```python
from build123d import *

# Parameters (mm, degrees)
SKETCH1_W                = 240
SKETCH1_H                = 151
BOSS_EXTRUDE1_DEPTH      = 5
SKETCH5_R                = 2
CUT_EXTRUDE1_DEPTH       = 5
SKETCH6_R                = 4
SKETCH6_R_2              = 2
BOSS_EXTRUDE2_DEPTH      = 5
CUT_EXTRUDE2_DEPTH       = 5
SKETCH8_W                = 30
SKETCH8_H                = 12.5
CUT_EXTRUDE3_DEPTH       = 5
SKETCH9_W                = 59
SKETCH9_H                = 121
CUT_EXTRUDE4_DEPTH       = 5
SKETCH12_W               = 18
SKETCH12_H               = 40
CUT_EXTRUDE7_DEPTH       = 10
SKETCH15_R               = 2
CUT_EXTRUDE9_DEPTH       = 5
SKETCH16_W               = 5.2
SKETCH16_H               = 20.2
CUT_EXTRUDE10_DEPTH      = 5
CUT_EXTRUDE11_DEPTH      = 10
CUT_EXTRUDE13_DEPTH      = 143.667445481
CUT_EXTRUDE13_DEPTH_BACK = 10
SKETCH23_R               = 2
CUT_EXTRUDE16_DEPTH      = 5
SKETCH24_R               = 4
SKETCH24_R_2             = 2
BOSS_EXTRUDE4_DEPTH      = 5
CUT_EXTRUDE19_DEPTH      = 10
SKETCH32_W               = 4
SKETCH32_H               = 30
SKETCH32_H_2             = 15
BOSS_EXTRUDE6_DEPTH      = 5
FILLET1_R                = 5
FILLET2_R                = 2
CUT_EXTRUDE22_DEPTH      = 5
SKETCH37_R               = 2
CUT_EXTRUDE25_DEPTH      = 10
SKETCH38_R               = 2
CUT_EXTRUDE26_DEPTH      = 10
CUT_EXTRUDE29_DEPTH      = 10
SKETCH43_R               = 2
CUT_EXTRUDE30_DEPTH      = 10
SKETCH44_R               = 4
SKETCH44_R_2             = 2
BOSS_EXTRUDE7_DEPTH      = 5
CUT_EXTRUDE31_DEPTH      = 10
CUT_EXTRUDE32_DEPTH      = 10
SKETCH47_R               = 2
CUT_EXTRUDE33_DEPTH      = 10
SKETCH48_W               = 15
SKETCH48_H               = 5
CUT_EXTRUDE34_DEPTH      = 5


with BuildPart() as part:
    # Sketch1 → Boss-Extrude1 (new body)
    with BuildSketch(Plane.XY):
        Rectangle(SKETCH1_W, SKETCH1_H)
    extrude(amount=BOSS_EXTRUDE1_DEPTH)

    # Sketch5 → Cut-Extrude1 (cut)
    with BuildSketch(Plane(origin=(0, 0, 0), x_dir=(-1, 0, 0), z_dir=(0, 0, -1))):
        with Locations((35.2, -73)):
            Circle(SKETCH5_R)
        with Locations((79.8, -73)):
            Circle(SKETCH5_R)
        with Locations((22.5, -65.3)):
            Circle(SKETCH5_R)
        with Locations(Location((22.5, -20.7, 0), (0, 0, 180))):
            Circle(SKETCH5_R)
        with Locations(Location((79.8, -13, 0), (0, 0, 180))):
            Circle(SKETCH5_R)
        with Locations(Location((35.2, -13, 0), (0, 0, 180))):
            Circle(SKETCH5_R)
    extrude(amount=-CUT_EXTRUDE1_DEPTH, mode=Mode.SUBTRACT)

    # Sketch6 → Boss-Extrude2 (add)
    # profile 1 of 2: a face of its own
    with BuildSketch(Plane(origin=(0, 0, 0), x_dir=(-1, 0, 0), z_dir=(0, 0, -1))):
        with Locations((35.2, -73)):
            Circle(SKETCH6_R)
        with Locations((35.2, -73)):
            Circle(SKETCH6_R_2, mode=Mode.SUBTRACT)
    # profile 2 of 2: a face of its own
    with BuildSketch(Plane(origin=(0, 0, 0), x_dir=(-1, 0, 0), z_dir=(0, 0, -1))):
        with Locations((79.8, -73)):
            Circle(SKETCH6_R)
        with Locations((79.8, -73)):
            Circle(SKETCH6_R_2, mode=Mode.SUBTRACT)
    extrude(amount=-BOSS_EXTRUDE2_DEPTH)

    # Sketch7 → Cut-Extrude2 (cut)
    with BuildSketch(Plane(origin=(0, 0, 0), x_dir=(-1, 0, 0), z_dir=(0, 0, -1))):
        with BuildLine():
            Line((120, -63), (43.5, -63))
            ThreePointArc((43.5, -63), (23.5, -43), (43.5, -23))
            Line((43.5, -23), (120, -23))
            Line((120, -23), (120, -63))
        make_face()
    extrude(amount=-CUT_EXTRUDE2_DEPTH, mode=Mode.SUBTRACT)

    # Sketch8 → Cut-Extrude3 (cut)
    with BuildSketch(Plane(origin=(0, 0, 0), x_dir=(-1, 0, 0), z_dir=(0, 0, -1))):
        with Locations((105, -69.25)):
            Rectangle(SKETCH8_W, SKETCH8_H)
    extrude(amount=-CUT_EXTRUDE3_DEPTH, mode=Mode.SUBTRACT)

    # Sketch9 → Cut-Extrude4 (cut)
    with BuildSketch(Plane(origin=(0, 0, 0), x_dir=(-1, 0, 0), z_dir=(0, 0, -1))):
        with Locations((-90.5, -15)):
            Rectangle(SKETCH9_W, SKETCH9_H)
    extrude(amount=-CUT_EXTRUDE4_DEPTH, mode=Mode.SUBTRACT)

    # Sketch12 → Cut-Extrude7 (cut)
    with BuildSketch(Plane(origin=(0, 0, 0), x_dir=(-1, 0, 0), z_dir=(0, 0, -1))):
        with Locations((-3, 55.5)):
            Rectangle(SKETCH12_W, SKETCH12_H)
    extrude(amount=-CUT_EXTRUDE7_DEPTH, mode=Mode.SUBTRACT)

    # Sketch15 → Cut-Extrude9 (cut)
    with BuildSketch(Plane.XY.offset(5)):
        with Locations((-63.5, 68.3)):
            Circle(SKETCH15_R)
    extrude(amount=-CUT_EXTRUDE9_DEPTH, mode=Mode.SUBTRACT)

    # Sketch16 → Cut-Extrude10 (cut)
    with BuildSketch(Plane(origin=(0, 0, 0), x_dir=(-1, 0, 0), z_dir=(0, 0, -1))):
        with Locations((63.6, 35.6)):
            Rectangle(SKETCH16_W, SKETCH16_H)
    extrude(amount=-CUT_EXTRUDE10_DEPTH, mode=Mode.SUBTRACT)

    # Sketch18 → Cut-Extrude11 (cut)
    with BuildSketch(Plane(origin=(0, 0, 0), x_dir=(-1, 0, 0), z_dir=(0, 0, -1))):
        with BuildLine():
            Line((-2.007007892, 12.8501367), (-2.007007892, 2.8501367))
            ThreePointArc((-2.007007892, 2.8501367), (-9.507007892, -4.6498633), (-17.007007892, 2.8501367))
            Line((-17.007007892, 2.8501367), (-17.007007892, 12.8501367))
            ThreePointArc((-17.007007892, 12.8501367), (-9.507007892, 20.3501367), (-2.007007892, 12.8501367))
        make_face()
    extrude(amount=-CUT_EXTRUDE11_DEPTH, mode=Mode.SUBTRACT)

    # Sketch20 → Cut-Extrude13 (cut, two sides: drawn at the far end of the back side and taken through both)
    with BuildSketch(Plane(origin=(0, 0, 0), x_dir=(-1, 0, 0), z_dir=(0, 0, -1)).offset(-CUT_EXTRUDE13_DEPTH_BACK)):
        with BuildLine():
            ThreePointArc((-33.7955627, -69.5), (-42.0455627, -61.25), (-50.2955627, -69.5))
            Line((-50.2955627, -69.5), (-50.2955627, -75.5))
            Line((-50.2955627, -75.5), (-33.7955627, -75.5))
            Line((-33.7955627, -75.5), (-33.7955627, -69.5))
        make_face()
    extrude(amount=CUT_EXTRUDE13_DEPTH + CUT_EXTRUDE13_DEPTH_BACK, mode=Mode.SUBTRACT)

    # Sketch23 → Cut-Extrude16 (cut)
    with BuildSketch(Plane(origin=(0, 0, 0), x_dir=(-1, 0, 0), z_dir=(0, 0, -1))):
        with Locations((-107.8, 73)):
            Circle(SKETCH23_R)
        with Locations((-30.2, 73)):
            Circle(SKETCH23_R)
    extrude(amount=-CUT_EXTRUDE16_DEPTH, mode=Mode.SUBTRACT)

    # Sketch24 → Boss-Extrude4 (add)
    # profile 1 of 2: a face of its own
    with BuildSketch(Plane(origin=(0, 0, 0), x_dir=(-1, 0, 0), z_dir=(0, 0, -1))):
        with Locations((-107.8, 73)):
            Circle(SKETCH24_R)
        with Locations((-107.8, 73)):
            Circle(SKETCH24_R_2, mode=Mode.SUBTRACT)
    # profile 2 of 2: a face of its own
    with BuildSketch(Plane(origin=(0, 0, 0), x_dir=(-1, 0, 0), z_dir=(0, 0, -1))):
        with Locations((-30.2, 73)):
            Circle(SKETCH24_R)
        with Locations((-30.2, 73)):
            Circle(SKETCH24_R_2, mode=Mode.SUBTRACT)
    extrude(amount=-BOSS_EXTRUDE4_DEPTH)

    # Sketch30 → Cut-Extrude19 (cut)
    with BuildSketch(Plane(origin=(0, 0, 0), x_dir=(-1, 0, 0), z_dir=(0, 0, -1))):
        with BuildLine():
            Line((110, -19), (98, -19))
            ThreePointArc((98, -19), (92, -13), (98, -7))
            Line((98, -7), (110, -7))
            ThreePointArc((110, -7), (116, -13), (110, -19))
        make_face()
    extrude(amount=-CUT_EXTRUDE19_DEPTH, mode=Mode.SUBTRACT)

    # Sketch32 → Boss-Extrude6 (add)
    with BuildSketch(Plane(origin=(0, 0, 0), x_dir=(-1, 0, 0), z_dir=(0, 0, -1))):
        with Locations((122, 30.5)):
            Rectangle(SKETCH32_W, SKETCH32_H)
        with Locations((-122, 60.5)):
            Rectangle(SKETCH32_W, SKETCH32_H_2)
    extrude(amount=-BOSS_EXTRUDE6_DEPTH)

    # Fillet1
    fillet1_edges = [part.edges().sort_by_distance(p)[0] for p in [
        (61, 45.5, 2.5),
    ]]
    fillet(fillet1_edges, radius=FILLET1_R)

    # Fillet2
    fillet2_edges = [part.edges().sort_by_distance(p)[0] for p in [
        (12, 75.5, 2.5),
        (-6, 75.5, 2.5),
        (33.7955627, -75.5, 2.5),
        (50.2955627, -75.5, 2.5),
        (-90, -63, 2.5),
    ]]
    fillet(fillet2_edges, radius=FILLET2_R)

    # Sketch34 → Cut-Extrude22 (cut)
    with BuildSketch(Plane(origin=(0, 0, 0), x_dir=(-1, 0, 0), z_dir=(0, 0, -1))):
        Polygon((115, 58.736739195), (120, 58.736739195), (120, 63.136739195), (115, 63.136739195), (115, 64.636739195), (111.7, 64.636739195), (111.7, 63.136739195), (95, 63.136739195), (95, 58.736739195), (111.7, 58.736739195), (111.7, 57.236739195), (115, 57.236739195), align=None)
    extrude(amount=-CUT_EXTRUDE22_DEPTH, mode=Mode.SUBTRACT)

    # Sketch37 → Cut-Extrude25 (cut)
    with BuildSketch(Plane(origin=(0, 0, 0), x_dir=(-1, 0, 0), z_dir=(0, 0, -1))):
        with Locations((-30, -52.5)):
            Circle(SKETCH37_R)
    extrude(amount=-CUT_EXTRUDE25_DEPTH, mode=Mode.SUBTRACT)

    # Sketch38 → Cut-Extrude26 (cut)
    with BuildSketch(Plane(origin=(0, 0, 0), x_dir=(-1, 0, 0), z_dir=(0, 0, -1))):
        with Locations((5.115159436, 18.266698226)):
            Circle(SKETCH38_R)
    extrude(amount=-CUT_EXTRUDE26_DEPTH, mode=Mode.SUBTRACT)

    # Sketch42 → Cut-Extrude29 (cut)
    with BuildSketch(Plane(origin=(0, 0, 0), x_dir=(-1, 0, 0), z_dir=(0, 0, -1))):
        with BuildLine():
            Line((-52, -47.5), (-52, 2.5))
            ThreePointArc((-52, 2.5), (-42.236373755, 30.573885063), (-30, 3.486201934))
            Line((-30, 3.486201934), (-30, -47.5))
            Line((-30, -47.5), (-52, -47.5))
        make_face()
    extrude(amount=-CUT_EXTRUDE29_DEPTH, mode=Mode.SUBTRACT)

    # Sketch43 → Cut-Extrude30 (cut)
    with BuildSketch(Plane(origin=(0, 0, 0), x_dir=(-1, 0, 0), z_dir=(0, 0, -1))):
        with Locations((-58.5, 2.3)):
            Circle(SKETCH43_R)
        with Locations((-58.5, -63.3)):
            Circle(SKETCH43_R)
    extrude(amount=-CUT_EXTRUDE30_DEPTH, mode=Mode.SUBTRACT)

    # Sketch44 → Boss-Extrude7 (add)
    # profile 1 of 2: a face of its own
    with BuildSketch(Plane(origin=(0, 0, 0), x_dir=(-1, 0, 0), z_dir=(0, 0, -1))):
        with Locations((-58.5, 2.3)):
            Circle(SKETCH44_R)
        with Locations((-58.5, 2.3)):
            Circle(SKETCH44_R_2, mode=Mode.SUBTRACT)
    # profile 2 of 2: a face of its own
    with BuildSketch(Plane(origin=(0, 0, 0), x_dir=(-1, 0, 0), z_dir=(0, 0, -1))):
        with Locations((-58.5, -63.3)):
            Circle(SKETCH44_R)
        with Locations((-58.5, -63.3)):
            Circle(SKETCH44_R_2, mode=Mode.SUBTRACT)
    extrude(amount=-BOSS_EXTRUDE7_DEPTH)

    # Sketch45 → Cut-Extrude31 (cut)
    with BuildSketch(Plane(origin=(0, 0, 0), x_dir=(-1, 0, 0), z_dir=(0, 0, -1))):
        with BuildLine():
            Line((23, 60.5), (23, 50.5))
            ThreePointArc((23, 50.5), (18, 45.5), (13, 50.5))
            Line((13, 50.5), (13, 60.5))
            ThreePointArc((13, 60.5), (18, 65.5), (23, 60.5))
        make_face()
    extrude(amount=-CUT_EXTRUDE31_DEPTH, mode=Mode.SUBTRACT)

    # Sketch46 → Cut-Extrude32 (cut)
    with BuildSketch(Plane(origin=(0, 0, 0), x_dir=(-1, 0, 0), z_dir=(0, 0, -1))):
        with BuildLine():
            Line((-46, 50), (-36, 50))
            ThreePointArc((-36, 50), (-29, 43), (-36, 36))
            Line((-36, 36), (-46, 36))
            ThreePointArc((-46, 36), (-53, 43), (-46, 50))
        make_face()
    extrude(amount=-CUT_EXTRUDE32_DEPTH, mode=Mode.SUBTRACT)

    # Sketch47 → Cut-Extrude33 (cut)
    with BuildSketch(Plane(origin=(0, 0, 0), x_dir=(-1, 0, 0), z_dir=(0, 0, -1))):
        with Locations((-90, 50.5)):
            Circle(SKETCH47_R)
    extrude(amount=-CUT_EXTRUDE33_DEPTH, mode=Mode.SUBTRACT)

    # Sketch48 → Cut-Extrude34 (cut)
    with BuildSketch(Plane(origin=(0, 0, 0), x_dir=(-1, 0, 0), z_dir=(0, 0, -1))):
        with Locations((93, 73)):
            Rectangle(SKETCH48_W, SKETCH48_H)
    extrude(amount=-CUT_EXTRUDE34_DEPTH, mode=Mode.SUBTRACT)


solid = part.part
```
Work out the finished part from the listing and answer in its coordinate system (mm). A direction names the side the tool comes from. Give positions to 0.01 mm unless a question says otherwise; leave off trailing zeros. Order: outer loops, then holes, each group sorted by start corner. A loop starts at its lowest first (then second) coordinate and runs counter-clockwise, first axis right, second up. Notation, with made-up numbers: (-23.75, 86.5) - (34.25, 86.5) arc R10 ccw to (34.25, 97.5) - close; hole circle Ø6 at (-37.5, 52). An arc over 180 degrees is marked (long way). One line per item, written item: value. Start each with the question number.
1. For a pull along Y with two mould halves and no side action, classify faces 1 (the face through (-58, -75.5, 2)), 2 (the face through (-47, 75.5, 2)), 3 (the face through (-90, -70, 2)), 4 (the face through (42.77, 30.54, 2.46)) as released by +Y, released by -Y, zero draft, split by the parting line, or undercut.
2. Section B-B, the plane x = -103.5 is taken. Write down the section's boundary in (y, z).
3. Consider line 1 (X direction, y = 2, z = 1.9); line 2 (X direction, y = -13, z = 2.05); line 3 (X direction, y = 57, z = 3.1). Determine where each line is inside the solid, lowest interval first.
4. Which of the six approach directions +Z, -Z, +X, -X, +Y, -Y give full straight-line access (tool end or side, diameter ignored) to faces 5 (the face through (9.34, -4.65, 2.46)), 6 (the face through (-120, -4, 2)), 7 (the face through (115, 75.5, 2)), 8 (the face through (-93, 70.5, 2))?
5. Each of these flat-tipped pins is pushed along its axis until it touches: pin 1 Ø1.2 at (x, z) = (122.5, 3) entering from -Y; pin 2 Ø1.5 at (y, z) = (-70.5, 2.5) entering from +X; pin 3 Ø1.7 at (y, z) = (63.5, 1.5) entering from -X. Where does it stop, or does it pass through?
6. Section D-D, the plane x = 80 is taken. Write down the section's boundary in (y, z).
7. Section A-A, the plane y = -43 is taken. Write down the section's boundary in (x, z), then the cut area to 4 significant figures.
8. Section C-C, the plane z = 3.55 is taken. Count the separate pieces of the cut face and the enclosed holes in it, then the cut area to 3 significant figures.
Filled sheet:
1. face 1: released by -Y
1. face 2: released by +Y
1. face 3: zero draft
1. face 4: undercut
2. outline: (-23, 0) - (-19, 0) - (-19, 5) - (-23, 5) - close; (-7, 0) - (58.74, 0) - (58.74, 5) - (-7, 5) - close; (63.14, 0) - (75.5, 0) - (75.5, 5) - (63.14, 5) - close
3. line 1: -120 to 2.06, 16.96 to 30, 52 to 56.52, 60.48 to 62.49
3. line 2: -120 to -116, -92 to -81.8, -77.8 to -37.2, -33.2 to 30, 52 to 61
3. line 3: -120 to -23, -13 to -6, 12 to 124
4. face 5: +Z, -Z
4. face 6: +Z, -Z, -X, -Y
4. face 7: +Z, -Z, +X, +Y
4. face 8: +Z, -Z, +Y
5. pin 1: y = 53
5. pin 2: x = 61
5. pin 3: x = -120
6. outline: (45.5, 0) - (75.5, 0) - (75.5, 5) - (45.5, 5) - close
7. outline: (-23.5, 0) - (30, 0) - (30, 5) - (-23.5, 5) - close; (52, 0) - (61, 0) - (61, 5) - (52, 5) - close
7. area: 312.5 mm²
8. separate pieces: 1
8. enclosed holes: 20
8. area: 21,000 mm²
